from build123d import *

# Parameters (mm, degrees)
SKETCH_1_R      = 2.1
SKETCH_1_R_2    = 13.25
EXTRUDE_1_DEPTH = 3
FILLET_1_R      = 5
FILLET_2_R      = 5


with BuildPart() as part:
    # Sketch 1 → Extrude 1 (new body)
    with BuildSketch(Plane(origin=(0, 0, 0), x_dir=(1, 0, 0), z_dir=(0, 1, 0))):
        with BuildLine():
            Line((7.5, -73.5), (-18.109134325, -73.5))
            Line((-18.109134325, -73.5), (-21.426901174, -73.5))
            ThreePointArc((-21.426901174, -73.5), (-40, -83.3), (-58.573098826, -73.5))
            Line((-58.573098826, -73.5), (-61.890865675, -73.5))
            Line((-61.890865675, -73.5), (-87.5, -73.5))
            Line((-87.5, -73.5), (-87.5, 7.5))
            Line((-87.5, 7.5), (-40, 7.5))
            Line((-40, 7.5), (7.5, 7.5))
            Line((7.5, 7.5), (7.5, -73.5))
        make_face()
        with Locations(Location((0, 0, 0), (0, 0, 270))):
            Circle(SKETCH_1_R, mode=Mode.SUBTRACT)
        with Locations(Location((0, -66, 0), (0, 0, 270))):
            Circle(SKETCH_1_R, mode=Mode.SUBTRACT)
        with Locations(Location((-27.625631329, -48.425631329, 0), (0, 0, 270))):
            Circle(SKETCH_1_R, mode=Mode.SUBTRACT)
        with Locations(Location((-40, -60.8, 0), (0, 0, 270))):
            Circle(SKETCH_1_R_2, mode=Mode.SUBTRACT)
        with Locations(Location((-27.625631329, -73.174368671, 0), (0, 0, 270))):
            Circle(SKETCH_1_R, mode=Mode.SUBTRACT)
        with Locations(Location((-52.374368671, -73.174368671, 0), (0, 0, 270))):
            Circle(SKETCH_1_R, mode=Mode.SUBTRACT)
        with Locations(Location((-52.374368671, -48.425631329, 0), (0, 0, 270))):
            Circle(SKETCH_1_R, mode=Mode.SUBTRACT)
        with Locations(Location((-80, -66, 0), (0, 0, 270))):
            Circle(SKETCH_1_R, mode=Mode.SUBTRACT)
        with Locations(Location((-80, 0, 0), (0, 0, 270))):
            Circle(SKETCH_1_R, mode=Mode.SUBTRACT)
        with BuildLine():
            Line((-7.5, -53.5), (-7.5, -7.5))
            Line((-7.5, -7.5), (-30, -7.5))
            Line((-30, -7.5), (-30, -40.644355629))
            ThreePointArc((-30, -40.644355629), (-23.089317494, -45.958207076), (-18.717143049, -53.5))
            Line((-18.717143049, -53.5), (-7.5, -53.5))
        make_face(mode=Mode.SUBTRACT)
        with BuildLine():
            Line((-72.5, -7.5), (-50, -7.5))
            Line((-50, -7.5), (-50, -40.644355629))
            ThreePointArc((-50, -40.644355629), (-56.910682506, -45.958207076), (-61.282856951, -53.5))
            Line((-61.282856951, -53.5), (-72.5, -53.5))
            Line((-72.5, -53.5), (-72.5, -7.5))
        make_face(mode=Mode.SUBTRACT)
    extrude(amount=EXTRUDE_1_DEPTH)

    # Fillet 1
    fillet_1_edges = [part.edges().sort_by_distance(p)[0] for p in [
        (-50, 1.5, 7.5),
        (-72.5, 1.5, 7.5),
        (-72.5, 1.5, 53.5),
        (-61.282856951, 1.5, 53.5),
        (-50, 1.5, 40.644355629),
        (-7.5, 1.5, 53.5),
        (-7.5, 1.5, 7.5),
        (-30, 1.5, 7.5),
        (-30, 1.5, 40.644355629),
        (-18.717143049, 1.5, 53.5),
    ]]
    fillet(fillet_1_edges, radius=FILLET_1_R)

    # Fillet 2
    fillet_2_edges = [part.edges().sort_by_distance(p)[0] for p in [
        (-87.5, 1.5, 73.5),
        (-87.5, 1.5, -7.5),
        (7.5, 1.5, -7.5),
        (7.5, 1.5, 73.5),
        (-21.426901174, 1.5, 73.5),
        (-58.573098826, 1.5, 73.5),
    ]]
    fillet(fillet_2_edges, radius=FILLET_2_R)


solid = part.part
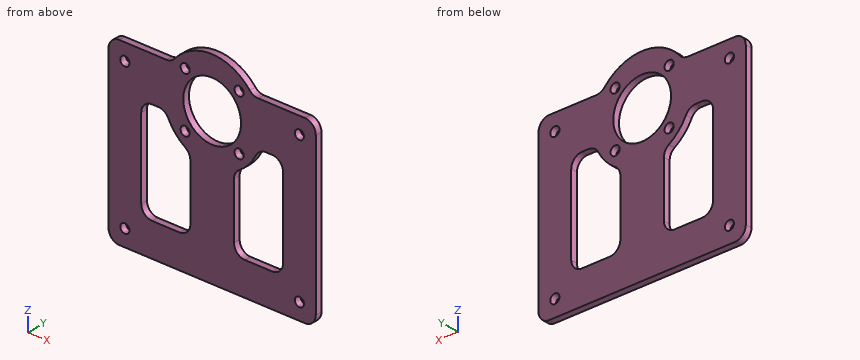
Check sheet for the modelled part. Datum: model origin and axes. Units: mm. Give positions to 0.01 mm unless a question says otherwise; leave off trailing zeros. Loops run counter-clockwise (first coordinate to the right, second up) from the corner with the lowest first, then second, coordinate; pieces in that order, holes last. Notation, with made-up numbers: M 23,17 L 71,17 A31 ccw 71,47 Z; hole C -29,89.25 d3. An arc over 180 degrees is marked long. Use a Markdown table: item, result. Add a question column.
Q1. Sectioned sample at D-D, the plane y = 1.85. Give the number of separate pieces and of enclosed holes in the cut face, then the cut area to 3 significant figures.
Q2. Sectioned sample at C-C, the plane z = 60.8. Record the cut outline in (x, y), then the cut area to 4 significant figures.
Q3. Sectioned sample at B-B, the plane z = 25. Record the cut outline in (x, y).
Q4. Scan lines: line 1 along X through (y, z) = (1.85, 0); line 2 along X through (y, z) = (2.05, 36); line 3 along X through (y, z) = (2.2, 60.8). Record each from-to range of solid material in increasing order. Write a range as [from, to].
Q5. Sectioned sample at A-A, the plane x = 0. Record the cut outline in (y, z), then the cut area to 3 significant figures.
Verdict:
| question | item | result |
|---|---|---|
| 1 | separate pieces | 1 |
| 1 | enclosed holes | 11 |
| 1 | area | 5,420 mm^2 |
| 2 | outline | M -87.5,0 L -53.25,0 L -53.25,3 L -87.5,3 Z; M -26.75,0 L 7.5,0 L 7.5,3 L -26.75,3 Z |
| 2 | area | 205.5 mm^2 |
| 3 | outline | M -87.5,0 L -72.5,0 L -72.5,3 L -87.5,3 Z; M -50,0 L -30,0 L -30,3 L -50,3 Z; M -7.5,0 L 7.5,0 L 7.5,3 L -7.5,3 Z |
| 4 | line 1 | [-87.5, -82.1], [-77.9, -2.1], [2.1, 7.5] |
| 4 | line 2 | [-87.5, -72.5], [-50, -30], [-7.5, 7.5] |
| 4 | line 3 | [-87.5, -53.25], [-26.75, 7.5] |
| 5 | outline | M 0,-7.5 L 3,-7.5 L 3,-2.1 L 0,-2.1 Z; M 0,2.1 L 3,2.1 L 3,63.9 L 0,63.9 Z; M 0,68.1 L 3,68.1 L 3,73.5 L 0,73.5 Z |
| 5 | area | 218 mm^2 |
